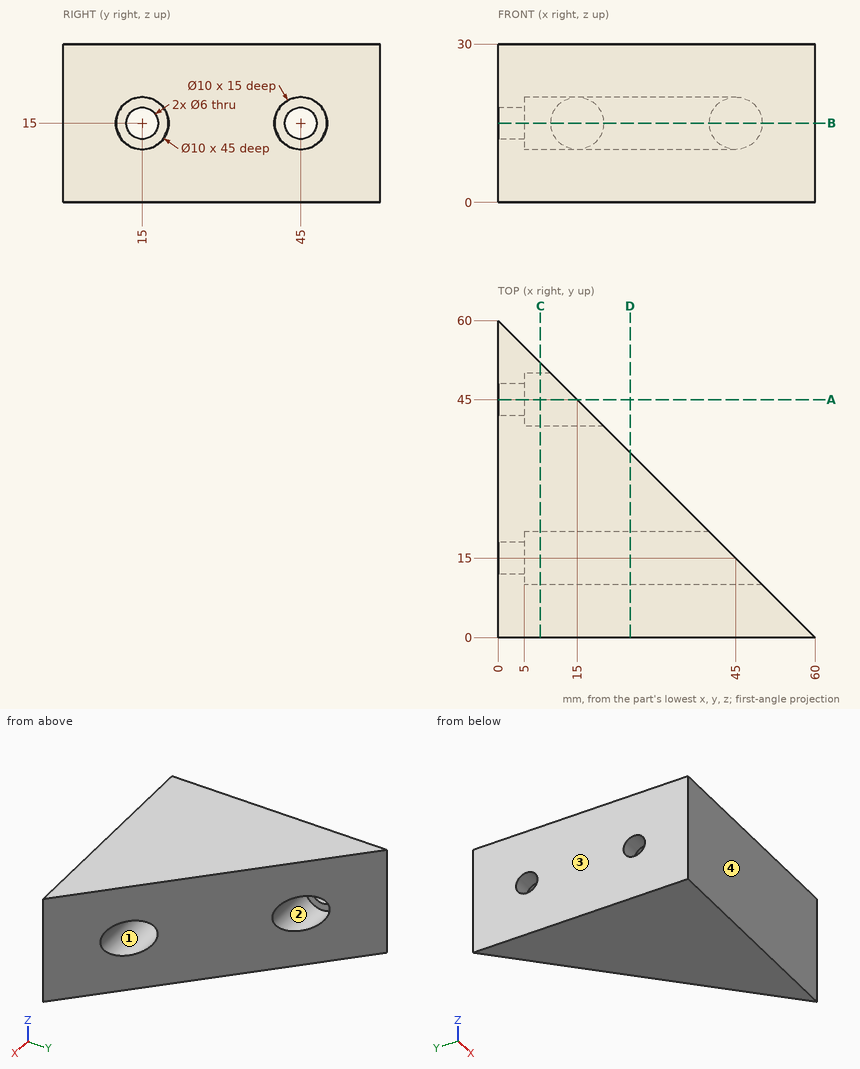
For this review, use the dimensioned drawing (mm, ordinates from the lowest corner) and the shaded views. Coordinates: 2 decimals unless noted, no trailing zeros. Loops run counter-clockwise (first coordinate to the right, second up) from the corner with the lowest first, then second, coordinate; pieces in that order, holes last. Notation, with made-up numbers: (66, -25.5) -> (120, -25.5) arc R26 ccw to (120, 3.5) -> close; hole circle Ø10 at (-2.75, 30.25). An arc over 180 degrees is marked (long way). Use a Markdown table: item, result. Add a question column.
1. Clearance check with flat-ended pins moving along their axes: pin 1 Ø11 at (y, z) = (13.5, 13) entering from +X; pin 2 Ø3 at (y, z) = (44.5, 14) entering from +X; pin 3 Ø12 at (y, z) = (37.5, 15.5) entering from +X; pin 4 Ø4 at (x, z) = (50.5, 11.5) entering from +Y. State where each tip first meets the part, or that it passes through.
2. To check wall thickness, follow line 1 (Y direction, x = 1.25, z = 15); line 2 (Z direction, x = 24.5, y = 11); line 3 (Y direction, x = 19, z = 15). State the ranges of each line that lie inside material, in increasing order.
3. Add section B-B on z = 15. Write out the cut boundary in (x, y).
4. Add section D-D on x = 25. Write out the cut boundary in (y, z).
5. Add section C-C on x = 8. Write out the cut boundary in (y, z).
6. Draft analysis for pull direction Y (two halves, no side actions). For the marked faces 1, 2, 3 and 4, state which applies: pulls with the +Y half, pulls with the -Y half, needs draft (parallel to the pull), parting line crosses it, or undercut.
7. Add section A-A on y = 45. Write out the cut boundary in (x, z).
Returned:
| question | item | result |
|---|---|---|
| 1 | pin 1 | stops at x = 52 |
| 1 | pin 2 | passes through |
| 1 | pin 3 | stops at x = 28.5 |
| 1 | pin 4 | stops at y = 11.5 |
| 2 | line 1 | y = 0 to 12, 18 to 42, 48 to 58.75 |
| 2 | line 2 | z = 0 to 12, 18 to 30 |
| 2 | line 3 | y = 0 to 10, 20 to 40 |
| 3 | outline | (0, 0) -> (60, 0) -> (50, 10) -> (5, 10) -> (5, 12) -> (0, 12) -> close; (0, 18) -> (5, 18) -> (5, 20) -> (40, 20) -> (20, 40) -> (5, 40) -> (5, 42) -> (0, 42) -> close; (0, 48) -> (5, 48) -> (5, 50) -> (10, 50) -> (0, 60) -> close |
| 4 | outline | (0, 0) -> (35, 0) -> (35, 30) -> (0, 30) -> close; hole circle Ø10 at (15, 15) |
| 5 | outline | (0, 0) -> (52, 0) -> (52, 30) -> (0, 30) -> close; hole circle Ø10 at (15, 15); hole circle Ø10 at (45, 15) |
| 6 | face 1 | undercut |
| 6 | face 2 | undercut |
| 6 | face 3 | needs draft |
| 6 | face 4 | pulls with the -Y half |
| 7 | outline | (0, 0) -> (15, 0) -> (15, 10) -> (5, 10) -> (5, 12) -> (0, 12) -> close; (0, 18) -> (5, 18) -> (5, 20) -> (15, 20) -> (15, 30) -> (0, 30) -> close |
